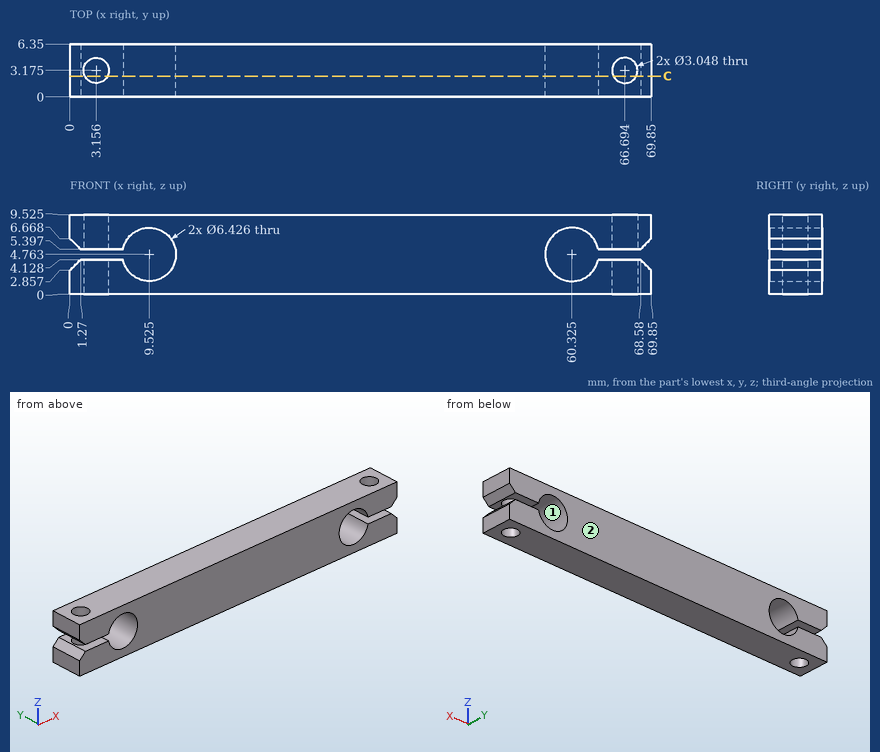
Part print with two shaded views. Sizes in mm from the minimum x, y, z corner. Round coordinates to 2 decimals unless told otherwise and drop trailing zeros. Use CSV: the item, a comma, the result in double quotes. Start each with the question number.
(1) Cut at C-C on y = 2.5. State how many separate pieces and enclosed holes the cut face has, then the cut area to 3 significant figures.
(2) Drill centre lines: probe 1 along Z at (x, y) = (5, 2.75) (1 decimal); probe 2 along X at (y, z) = (0.5, 5); probe 3 along X at (y, z) = (1.25, 3.75) (1 decimal). Where is each one in solid material? Low to high.
(3) Mould opens along X. For the marked faces 1 and 2 say: +X half, -X half, draft (parallel to the pull), parting line (faces both ways), or undercut.
(4) Flat gauge pin, fed straight in: P1, Ø5, axis at x = 9.52, z = 4.76, coming from the +Y side. Where does the tip first touch, or does it go through?
Findings:
1,separate pieces,"5"
1,enclosed holes,"0"
1,area,"536 mm^2"
2,probe 1,"z = 0 to 4.1, 5.4 to 9.5"
2,probe 2,"x = 12.73 to 57.12"
2,probe 3,"x = 0.9 to 6.5, 12.6 to 57.3, 63.4 to 69"
3,face 1,"undercut"
3,face 2,"draft"
4,P1,"passes through"
